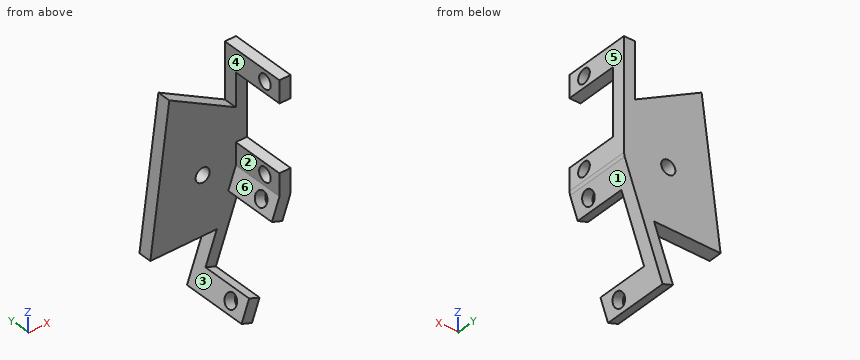
from build123d import *

# Parameters (mm, degrees)
BOSS_EXTRUDE1_DEPTH = 15
SKETCH5_R           = 1.6
SKETCH5_W           = 15
SKETCH5_H           = 12
CUT_EXTRUDE4_DEPTH  = 15
SKETCH8_R           = 1.6
SKETCH8_W           = 15
SKETCH8_H           = 12.119225193
CUT_EXTRUDE5_DEPTH  = 15
SKETCH6_R           = 1.6
BOSS_EXTRUDE8_DEPTH = 3


with BuildPart() as part:
    # Sketch1 → Boss-Extrude1 (new body)
    with BuildSketch(Plane(origin=(0, 0, 0), x_dir=(1, 0, 0), z_dir=(0, 1, 0))):
        Polygon((-0.46984631, -0.171010072), (-0.46984631, -25.171010072), (-2.96984631, -25.171010072), (-2.96984631, -0.171010072), (-11.520349894, 23.321305448), (-9.171118342, 24.176355806), (-0.620614758, 0.684040287), align=None)
    extrude(amount=-BOSS_EXTRUDE1_DEPTH)

    # Sketch5 → Cut-Extrude4 (cut)
    with BuildSketch(Plane(origin=(-0.46984631, 0, 0), x_dir=(0, 0, -1), z_dir=(1, 0, 0))):
        with Locations((-22.671010072, -11)):
            Circle(SKETCH5_R)
        with Locations((-2.671010072, -11)):
            Circle(SKETCH5_R)
        with Locations((-12.671010072, -9)):
            Rectangle(SKETCH5_W, SKETCH5_H)
    extrude(amount=-CUT_EXTRUDE4_DEPTH, mode=Mode.SUBTRACT)

    # Sketch8 → Cut-Extrude5 (cut)
    with BuildSketch(Plane(origin=(-0.328170312, 0, 0.119444225), x_dir=(-0.342020143, 0, -0.939692621), z_dir=(0.939692621, 0, -0.342020143))):
        with Locations((3.355050358, -11)):
            Circle(SKETCH8_R)
        with Locations((23.355050358, -11)):
            Circle(SKETCH8_R)
        with Locations((13.355050358, -9.059612596)):
            Rectangle(SKETCH8_W, SKETCH8_H)
    extrude(amount=-CUT_EXTRUDE5_DEPTH, mode=Mode.SUBTRACT)

    # Sketch6 → Boss-Extrude8 (add)
    with BuildSketch(Plane(origin=(0, 0, 0), x_dir=(1, 0, 0), z_dir=(0, 1, 0))):
        Polygon((-7.245098102, 11.575147688), (-22.245098102, 11.575147688), (-17.96984631, -21.01652559), (-2.96984631, -12.671010072), (-0.46984631, -0.171010072), (-0.620614758, 0.684040287), align=None)
        with Locations((-10.452336242, -1.490374929)):
            Circle(SKETCH6_R, mode=Mode.SUBTRACT)
    extrude(amount=-BOSS_EXTRUDE8_DEPTH)


solid = part.part
Design review of the part built by this model. Coordinates are the model's own, in mm. Face numbers are marked on the shaded views. A direction names the side the tool comes from. Round coordinates to 2 decimals unless told otherwise and drop trailing zeros. Write each loop counter-clockwise with the first axis right and the second up, starting at its lowest first coordinate (ties: lowest second). Pieces come first, ordered by that corner, then holes. Notation, with made-up numbers: (-30, 46) - (-10, 46) arc R34 ccw to (-10, 77) - close; hole circle Ø1 at (15, 55). An arc over 180 degrees is marked (long way). Return JSON: item names as keys, results as strings. Group by question number.
Item 1: For probe 1 along Y at (x, z) = (-12.5, -4); probe 2 along X at (y, z) = (-1.5, 0.5); probe 3 along X at (y, z) = (-0.5, 2), list the stretches that pass through material, from the lowest coordinate up. Write a range as [from, to].
Item 2: Machinability: for the marked faces 1, 2 and 3, which of the approach directions +Z, -Z, +X, -X, +Y, -Y give a long, thin tool a straight path to every point of the face, cutting with its end or side? Answer none if there is none.
Item 3: Insertion check: P1, Ø10, axis at x = -13, z = -7.5, coming from the -Y side; P2, Ø1.5, axis at y = -9, z = 2, coming from the -X side; P3, Ø2, axis at x = -10.5, y = -5, coming from the +Z side. Each pin has a flat end and moves straight along its axis. Give the tip position at first contact, or say it passes through.
Item 4: We need section C-C on x = -12.75. Write out the cut boundary in (y, z).
Item 5: We need section A-A on y = -5. Write out the cut boundary in (x, z).
Item 6: The part is to be moulded in two halves that separate along X. For the marked faces 4, 5 and 6, say which applies: pulls with the +X half, pulls with the -X half, needs draft (parallel to the pull), parting line crosses it, or undercut.
Item 7: We need section D-D on z = 6.5. Write out the cut boundary in (x, y).
Item 8: We need section B-B on y = -11. Give the number of separate pieces and of enclosed holes in the cut face, and give its area (3 significant figures).
Model answer:
{
 "1": {"probe 1": "y = [-3, 0]", "probe 2": "x = [-20.66, -11.71], [-9.2, -0.47]", "probe 3": "x = [-20.46, -11.97], [-8.94, -0.47]"},
 "2": {"face 1": "-Z, +X, +Y, -Y", "face 2": "+Z, -X, -Y", "face 3": "-X, +Y, -Y"},
 "3": {"P1": "stops at y = -3", "P2": "stops at x = -2.97", "P3": "stops at z = -18.62"},
 "4": {"outline": "(-3, -11.58) - (0, -11.58) - (0, 18.11) - (-3, 18.11) - close"},
 "5": {"outline": "(-11.52, -23.32) - (-9.17, -24.18) - (-7.46, -19.48) - (-9.81, -18.62) - close; (-4.68, -4.53) - (-2.33, -5.38) - (-0.62, -0.68) - (-0.47, 0.17) - (-0.47, 5.17) - (-2.97, 5.17) - (-2.97, 0.17) - close; (-2.97, 20.17) - (-0.47, 20.17) - (-0.47, 25.17) - (-2.97, 25.17) - close"},
 "6": {"face 4": "undercut", "face 5": "pulls with the +X half", "face 6": "pulls with the -X half"},
 "7": {"outline": "(-19.87, -3) - (-0.47, -3) - (-0.47, 0) - (-19.87, 0) - close"},
 "8": {"separate pieces": "7", "enclosed holes": "0", "area": "19.1 mm²"}
}
